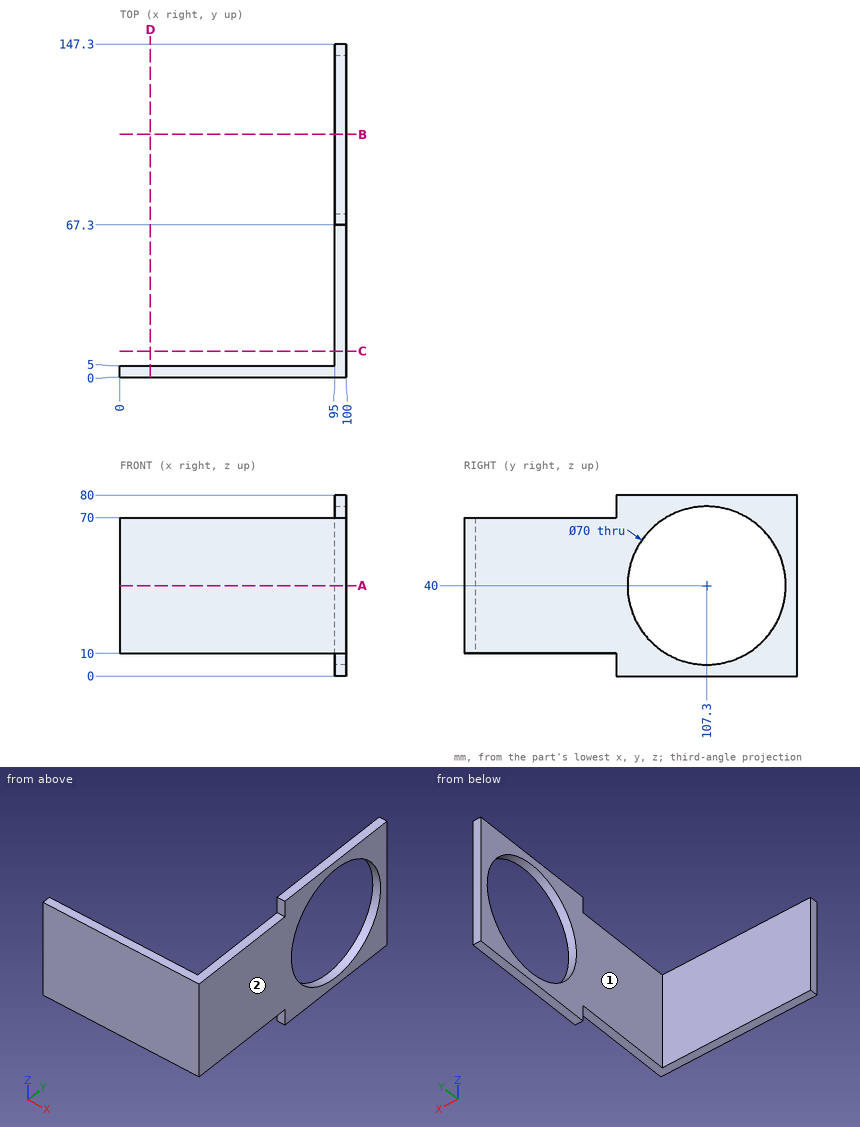
Input: dimensioned drawing with shaded views. Units: mm. Origin: part minimum x, y, z. A direction names the side the tool comes from. Coordinates: 2 decimals unless noted, no trailing zeros. Write each loop counter-clockwise with the first axis right and the second up, starting at its lowest first coordinate (ties: lowest second). Pieces come first, ordered by that corner, then holes. Notation, with made-up numbers: M -9.75,27 L 42.25,27 A28 ccw 42.25,57 Z; hole C 47,-36.75 d10. An arc over 180 degrees is marked long. Answer as a JSON object with one key per item and string values. Group by question number.
(1) Section A-A on z = 40. Output: boundary loops of the cut face in (x, y), plus the area to 4 significant figures.
(2) Section D-D on x = 13.5. Output: boundary loops of the cut face in (y, z), plus the area to 3 significant figures.
(3) Ray query, line 1 along Y through (x, z) = (97, 40); line 2 along Z through (x, y) = (96, 107); line 3 along X through (y, z) = (55, 65). Return the intervals inside material, ascending. Write a range as [from, to].
(4) Section C-C on y = 11.5. Output: boundary loops of the cut face in (x, z).
(5) Section B-B on y = 107.3. Output: boundary loops of the cut face in (x, z), plus the area to 3 significant figures.
(6) Set-up query: the marked faces 1 and 2. Return all of +Z, -Z, +X, -X, +Y, -Y with unobstructed straight access to the full face (end or side cutting, diameter ignored); none if empty.
(7) Contact query for flat-ended pins moving along their axis: P1, Ø1.5, axis at y = 45.5, z = 56, coming from the -X side; P2, Ø1.5, axis at x = 98.5, z = 5.5, coming from the -Y side; P3, Ø2, axis at x = 46, z = 19, coming from the +Y side. Output: stop coordinate, or through.
Result set:
{
 "1": {"outline": "M 0,0 L 100,0 L 100,72.3 L 95,72.3 L 95,5 L 0,5 Z; M 95,142.3 L 100,142.3 L 100,147.3 L 95,147.3 Z", "area": "861.5 mm2"},
 "2": {"outline": "M 0,10 L 5,10 L 5,70 L 0,70 Z", "area": "300 mm2"},
 "3": {"line 1": "y = [0, 72.3], [142.3, 147.3]", "line 2": "z = [0, 5], [75, 80]", "line 3": "x = [95, 100]"},
 "4": {"outline": "M 95,10 L 100,10 L 100,70 L 95,70 Z"},
 "5": {"outline": "M 95,0 L 100,0 L 100,5 L 95,5 Z; M 95,75 L 100,75 L 100,80 L 95,80 Z", "area": "50.0 mm2"},
 "6": {"face 1": "+Z, -Z, -X, +Y", "face 2": "+Z, -Z, +X, +Y, -Y"},
 "7": {"P1": "stops at x = 95", "P2": "stops at y = 67.3", "P3": "stops at y = 5"}
}
